The model under review builds one solid part; all positions refer to its coordinate system, in mm. Face numbers are marked on the shaded views. A direction names the side the tool comes from. Give positions to 0.01 mm unless a question says otherwise; leave off trailing zeros. Write each loop counter-clockwise with the first axis right and the second up, starting at its lowest first coordinate (ties: lowest second). Pieces come first, ordered by that corner, then holes. Notation, with made-up numbers: (-6, 7.5) - (0, 7.5) arc R22 ccw to (0, 42.5) - close; hole circle Ø8 at (-30.75, 36.5). An arc over 180 degrees is marked (long way). Write item = value, one per line.
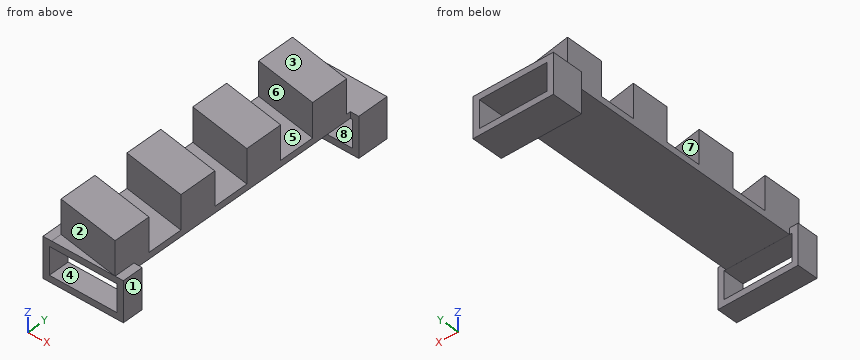
```python
from build123d import *

# Parameters (mm, degrees)
F0_W     = 30
F0_H     = 140
F1_DEPTH = 3
F3_DEPTH = 16
F4_W     = 3
F4_H     = 3
F4_W_2   = 1
F4_W_3   = 30
F4_W_4   = 32
F5_DEPTH = 15
F6_W     = 3
F6_H     = 3
F6_W_2   = 32
F7_DEPTH = 10


with BuildPart() as f1:
    # F0 (on Top) → F1 (new body)
    with BuildSketch(Plane.XY):
        with Locations((27.8885364532, 24.2495501014)):
            Rectangle(F0_W, F0_H)
    extrude(amount=F1_DEPTH)

    # F2 (on face) → F3 (join)
    with BuildSketch(Plane.XY.offset(3)):
        Polygon((42.8885364532, -27.7504498986), (12.8885364532, -22.7504498986), (12.8885364532, -40.7504498986), (42.8885364532, -45.7504498986), align=None)
        Polygon((12.8885364532, 12.2495501014), (12.8885364532, -5.7504498986), (42.8885364532, -10.7504498986), (42.8885364532, 7.2495501014), align=None)
        Polygon((12.8885364532, 47.2495501014), (12.8885364532, 29.2495501014), (42.8885364532, 24.2495501014), (42.8885364532, 42.2495501014), align=None)
        Polygon((12.8885364532, 82.2495501014), (12.8885364532, 64.2495501014), (42.8885364532, 59.2495501014), (42.8885364532, 77.2495501014), align=None)
    extrude(amount=F3_DEPTH)

    # F4 (on face) → F5 (join)
    with BuildSketch(Plane(origin=(0, 94.2495501014, 0), x_dir=(-1, 0, 0), z_dir=(0, 1, 0))):
        with Locations((-45.3885364532, 1.5)):
            Rectangle(F4_W, F4_H)
        with Locations((-43.3885364532, 1.5)):
            Rectangle(F4_W_2, F4_H)
        Polygon((-43.8885364532, 0), (-46.8885364532, 0), (-46.8885364532, -16), (-43.8885364532, -16), (-43.8885364532, -13), align=None)
        with Locations((-27.8885364532, 1.5)):
            Rectangle(F4_W_3, F4_H)
        with Locations((-27.8885364532, -14.5)):
            Rectangle(F4_W_4, F4_H)
        with Locations((-12.3885364532, 1.5)):
            Rectangle(F4_W_2, F4_H)
        Polygon((-11.8885364532, 0), (-11.8885364532, -13), (-11.8885364532, -16), (-8.8885364532, -16), (-8.8885364532, 0), align=None)
        with Locations((-10.3885364532, 1.5)):
            Rectangle(F4_W, F4_H)
    extrude(amount=-F5_DEPTH)

    # F6 (on face) → F7 (join)
    with BuildSketch(Plane.XZ.offset(45.7504498986)):
        with Locations((10.2999972403, 1.4885346591)):
            Rectangle(F6_W, F6_H)
        Polygon((11.7999972403, -0.0114653409), (8.7999972403, -0.0114653409), (8.7999972403, -16.0114653409), (11.7999972403, -16.0114653409), (11.7999972403, -13.0114653409), align=None)
        with Locations((27.7999972403, -14.5114653409)):
            Rectangle(F6_W_2, F6_H)
        Polygon((46.7999972403, -0.0114653409), (43.7999972403, -0.0114653409), (43.7999972403, -13.0114653409), (43.7999972403, -16.0114653409), (46.7999972403, -16.0114653409), align=None)
        with Locations((45.2999972403, 1.4885346591)):
            Rectangle(F6_W, F6_H)
        Polygon((12.8885364532, 2.9885346591), (11.7999972403, 2.9885346591), (11.7999972403, -0.0114653409), (43.7999972403, -0.0114653409), (43.7999972403, 2.9885346591), (42.8885364532, 2.9885346591), (42.8885364532, 0), (12.8885364532, 0), align=None)
    extrude(amount=-F7_DEPTH)


solid = f1.part
```
1. For line 1 (Y direction, x = 25.5, z = -13.5); line 2 (Z direction, x = 17, y = 83.5); line 3 (Y direction, x = 33, z = 4), list the stretches that pass through material, from the lowest coordinate up. Write a range as from..to.
Findings below:
line_1 = -45.75..-35.75, 79.25..94.25
line_2 = -16..-13, 0..3
line_3 = -44.1..-26.1, -9.1..8.9, 25.9..43.9, 60.9..78.9
2. Take a section at A-A on z = -7. Give the boundary of the cut face in (x, y), and give its area (3 significant figures).
Findings below:
outline = (8.8, -45.75) - (11.8, -45.75) - (11.8, -35.75) - (8.8, -35.75) - close; (8.89, 79.25) - (11.89, 79.25) - (11.89, 94.25) - (8.89, 94.25) - close; (43.8, -45.75) - (46.8, -45.75) - (46.8, -35.75) - (43.8, -35.75) - close; (43.89, 79.25) - (46.89, 79.25) - (46.89, 94.25) - (43.89, 94.25) - close
area = 150 mm²
3. Draft analysis for pull direction X (two halves, no side actions). For the marked faces 1, 2, 3 and 4, state which applies: +X half, -X half, draft (parallel to the pull), parting line (faces both ways), or undercut.
Findings below:
face_1 = +X half
face_2 = -X half
face_3 = draft
face_4 = undercut
4. Take a section at D-D on y = 27. Give the boundary of the cut face in (x, z), and give its area (3 significant figures).
Findings below:
outline = (12.89, 0) - (42.89, 0) - (42.89, 19) - (26.39, 19) - (26.39, 3) - (12.89, 3) - close
area = 354 mm²
5. Take a section at B-B on x = 33.5. Count the separate pieces of the cut face and the enclosed holes in it, and give its area (3 significant figures).
Findings below:
separate_pieces = 3
enclosed_holes = 0
area = 1,650 mm²
6. Take a section at C-C on z = 11. Give the boundary of the cut face in (x, y).
Findings below:
outline = (12.89, -40.75) - (42.89, -45.75) - (42.89, -27.75) - (12.89, -22.75) - close; (12.89, -5.75) - (42.89, -10.75) - (42.89, 7.25) - (12.89, 12.25) - close; (12.89, 29.25) - (42.89, 24.25) - (42.89, 42.25) - (12.89, 47.25) - close; (12.89, 64.25) - (42.89, 59.25) - (42.89, 77.25) - (12.89, 82.25) - close
7. Insertion check: P1, Ø14.5, axis at y = 85, z = -3.5, coming from the -X side; P2, Ø2, axis at x = 11, y = -43, coming from the +Z side; P3, Ø2, axis at y = 17.5, z = 5.5, coming from the -X side; P4, Ø11, axis at x = 28.5, y = 23, coming from the +Z side. Each pin has a flat end and moves straight along its axis. Give the tip position at first contact, or say it passes through.
Findings below:
P1 = 8.89
P2 = 2.99
P3 = through
P4 = 19
8. Machinability: for the marked faces 5, 6, 7 and 8, which of the approach directions +Z, -Z, +X, -X, +Y, -Y give a long, thin tool a straight path to every point of the face, cutting with its end or side? Answer none if there is none.
Findings below:
face_5 = +Z
face_6 = +Z, -X
face_7 = +Z, +X
face_8 = +Y, -Y
